Can you work these out from the model? Positions are in its coordinate system, mm. A direction names the side the tool comes from. Coordinates: 2 decimals unless noted, no trailing zeros. Order: outer loops, then holes, each group sorted by start corner. A loop starts at its lowest first (then second) coordinate and runs counter-clockwise, first axis right, second up. Notation, with made-up numbers: (17, -17.5) -> (56, -17.5) arc R22 ccw to (56, 19.5) -> close; hole circle Ø3 at (-39.5, 30.25). An arc over 180 degrees is marked (long way). Return JSON: item names as keys, results as strings. Group by question number.
1) If we section it at B-B, the plane y = 5: Please give me the cut outline in (x, z).
2) If we section it at A-A, the plane x = 5: Please give me the cut outline in (y, z).
3) If we section it at C-C, the plane z = 0.7: Please give me the cut outline in (x, y), then the cut area to 3 significant figures.
4) Thinking about a two-plate mould opening in X: for faces 3 (the cylindrical face through (5.54, 55.84, 1.97)), 4 (the flat face through (10, 10, 2)), 5 (the flat face through (0, 30, 2)), 6 (the flat face through (8, 30, 4)), which applies, +X half, -X half, draft (parallel to the pull), parting line (faces both ways), or undercut?
5) For faces 1 (the flat face through (15, 40, 2)), 2 (the cylindrical face through (11.203, 18.859, 1.972)), which set-ups out of +Z, -Z, +X, -X, +Y, -Y let a thin tool reach every point of the face, with its end or its side?
6) For pin 1 (1 mm diameter, centred on y = 8.5, z = 2, fed in from +X); pin 2 (1 mm diameter, centred on x = 15.5, z = 1.5, fed in from -Y); pin 3 (0.6 mm diameter, centred on x = 14.5, z = 1.5, fed in from +Y), each with a flat end and sliding along its axis, tell me the tip position at first contact or that it passes through.
7) If I drill on probe 1 along Y at (x, z) = (5, 1.1); probe 2 along X at (y, z) = (5, 0.95); probe 3 along X at (y, z) = (8, 3.3), over which ranges is the centre line in solid material (lowest first)? Write a range as from..to.
8) If we section it at D-D, the plane y = 45: Please give me the cut outline in (x, z).
from build123d import *

# Parameters (mm, degrees)
CYLINDER005_R     = 1
CYLINDER005_DEPTH = 20
ARRAY005_Y_COUNT  = 2
ARRAY005_Y_PITCH  = 50
BOX005_W          = 20
BOX005_H          = 20
BOX005_DEPTH      = 4
BOX004_W          = 10
BOX004_H          = 60
BOX004_DEPTH      = 4
FILLET_R          = 4
FILLET001_R       = 4


with BuildPart() as ear_screw_hole_fusion_array:
    # Cylinder005 → Cylinder005 (new body)
    with BuildSketch(Plane.XY.offset(40)):
        Circle(CYLINDER005_R)
    extrude(amount=CYLINDER005_DEPTH)

    # Array005 Y: ear screw hole fusion array ×2


with BuildPart() as ear_screw_hole_fusion_array_1:
    add(ear_screw_hole_fusion_array.part)
    with Locations(*[(0, i * ARRAY005_Y_PITCH, 0) for i in range(1, ARRAY005_Y_COUNT)]):
        add(ear_screw_hole_fusion_array.part)


with BuildPart() as ear_screw_hole_fusion_array_2:
    # Array005 placement: moved
    add(ear_screw_hole_fusion_array_1.part.moved(Location((5, 5, -40))))


with BuildPart() as mount_plate:
    # Box005 → Box005 (new body)
    with BuildSketch(Plane(origin=(0, 20, 0), x_dir=(1, 0, 0), z_dir=(0, 0, 1))):
        with Locations((10, 10)):
            Rectangle(BOX005_W, BOX005_H)
    extrude(amount=BOX005_DEPTH)


with BuildPart() as ear_mount_cut:
    # Box004 → Box004 (new body)
    with BuildSketch(Plane.XY):
        with Locations((5, 30)):
            Rectangle(BOX004_W, BOX004_H)
    extrude(amount=BOX004_DEPTH)

    # Fillet
    fillet_edges = [ear_mount_cut.edges().sort_by_distance(p)[0] for p in [
        (0, 0, 2),
        (0, 60, 2),
        (10, 0, 2),
        (10, 60, 2),
    ]]
    fillet(fillet_edges, radius=FILLET_R)

    # Fusion001: union mount plate
    add(mount_plate.part)

    # Fillet001
    fillet001_edges = [ear_mount_cut.edges().sort_by_distance(p)[0] for p in [
        (10, 20, 2),
        (10, 40, 2),
        (20, 40, 2),
        (20, 20, 2),
    ]]
    fillet(fillet001_edges, radius=FILLET001_R)

    # Cut023015002: cut ear screw hole fusion array
    add(ear_screw_hole_fusion_array_2.part, mode=Mode.SUBTRACT)


solid = ear_mount_cut.part
Result sheet:
{
 "1": {"outline": "(0, 0) -> (4, 0) -> (4, 4) -> (0, 4) -> close; (6, 0) -> (10, 0) -> (10, 4) -> (6, 4) -> close"},
 "2": {"outline": "(0, 0) -> (4, 0) -> (4, 4) -> (0, 4) -> close; (6, 0) -> (54, 0) -> (54, 4) -> (6, 4) -> close; (56, 0) -> (60, 0) -> (60, 4) -> (56, 4) -> close"},
 "3": {"outline": "(0, 4) arc R4 ccw to (4, 0) -> (6, 0) arc R4 ccw to (10, 4) -> (10, 16) arc R4 cw to (14, 20) -> (16, 20) arc R4 ccw to (20, 24) -> (20, 36) arc R4 ccw to (16, 40) -> (14, 40) arc R4 cw to (10, 44) -> (10, 56) arc R4 ccw to (6, 60) -> (4, 60) arc R4 ccw to (0, 56) -> close; hole circle Ø2 at (5, 5); hole circle Ø2 at (5, 55)", "area": "780 mm2"},
 "4": {"face 3": "undercut", "face 4": "+X half", "face 5": "-X half", "face 6": "draft"},
 "5": {"face 1": "+Z, -Z, +X, +Y", "face 2": "+Z, -Z, +X, -Y"},
 "6": {"pin 1": "stops at x = 10", "pin 2": "stops at y = 20", "pin 3": "stops at y = 40"},
 "7": {"probe 1": "y = 0..4, 6..54, 56..60", "probe 2": "x = 0..4, 6..10", "probe 3": "x = 0..10"},
 "8": {"outline": "(0, 0) -> (10, 0) -> (10, 4) -> (0, 4) -> close"}
}
